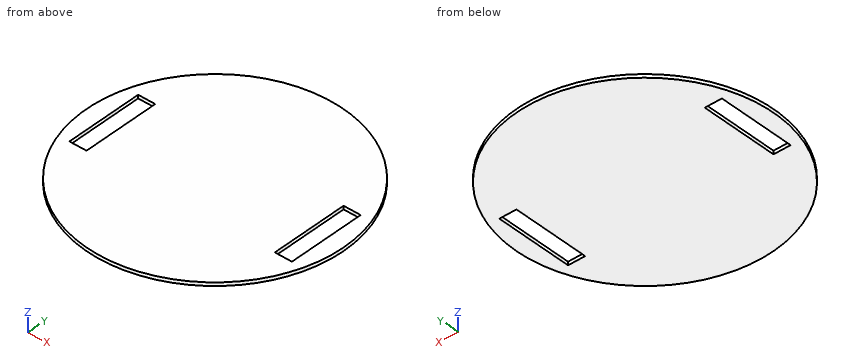
```python
from build123d import *

# Parameters (mm, degrees)
F0_R     = 75
F1_DEPTH = 2
F3_W     = 10
F3_H     = 22.5
F3_H_2   = 45
F4_DEPTH = 25


with BuildPart() as f1:
    # F0 (on Top) → F1 (new body)
    with BuildSketch(Plane.XY):
        Circle(F0_R)
    extrude(amount=F1_DEPTH)

    # F3 (on face) → F4 (cut)
    with BuildSketch(Plane.XY.offset(2)):
        with Locations((-60, -11.25)):
            Rectangle(F3_W, F3_H)
        with Locations((-60, 11.25)):
            Rectangle(F3_W, F3_H)
        with Locations((60, 0)):
            Rectangle(F3_W, F3_H_2)
    extrude(amount=-F4_DEPTH, mode=Mode.SUBTRACT)


solid = f1.part
```
Geometry check sheet. Reference: the model listing, model coordinates, mm. Coordinates: 2 decimals unless noted, no trailing zeros. Order: outer loops, then holes, each group sorted by start corner. A loop starts at its lowest first (then second) coordinate and runs counter-clockwise, first axis right, second up. Notation, with made-up numbers: (23, 60.25) - (33, 60.25) arc R16 ccw to (33, 84.25) - close; hole circle Ø1 at (75.5, 56). An arc over 180 degrees is marked (long way). Answer in a Markdown table with one row per item. Add a question column.
1. Section check D-D (x = 49). Enter the section's corners in (y, z), plus the area to 3 significant figures.
2. Material ranges on L1, parallel to X at y = -18.5, z = 0.9; L2, parallel to X at y = -19.5, z = 0.3; L3, parallel to Y at x = -64, z = 1.5, recorded low to high. Write a range as [from, to].
3. Gauge pin test, flat ends, axial feed: pin 1 Ø5 at (x, y) = (14.5, -37) entering from -Z; pin 2 Ø1 at (y, z) = (-3, 1) entering from -X; pin 3 Ø1 at (y, z) = (11, 1) entering from +X; pin 4 Ø6 at (x, y) = (-59, -52) entering from +Z. Record the tip position at first contact, or that the pin passes through.
4. Section check A-A (z = 0.6). Enter the section's corners in (x, y), plus the area to 3 significant figures.
5. Section check B-B (y = 0). Enter the section's corners in (x, z).
6. Section check C-C (y = -18). Enter the section's corners in (x, z).
Data:
| question | item | result |
|---|---|---|
| 1 | outline | (-56.78, 0) - (56.78, 0) - (56.78, 2) - (-56.78, 2) - close |
| 1 | area | 227 mm² |
| 2 | L1 | x = [-72.68, -65], [-55, 55], [65, 72.68] |
| 2 | L2 | x = [-72.42, -65], [-55, 55], [65, 72.42] |
| 2 | L3 | y = [-39.1, -22.5], [22.5, 39.1] |
| 3 | pin 1 | stops at z = 0 |
| 3 | pin 2 | stops at x = -74.96 |
| 3 | pin 3 | stops at x = 74.26 |
| 3 | pin 4 | passes through |
| 4 | outline | circle Ø150 at (0, 0); hole (-65, -22.5) - (-55, -22.5) - (-55, 22.5) - (-65, 22.5) - close; hole (55, -22.5) - (65, -22.5) - (65, 22.5) - (55, 22.5) - close |
| 4 | area | 16,800 mm² |
| 5 | outline | (-75, 0) - (-65, 0) - (-65, 2) - (-75, 2) - close; (-55, 0) - (55, 0) - (55, 2) - (-55, 2) - close; (65, 0) - (75, 0) - (75, 2) - (65, 2) - close |
| 6 | outline | (-72.81, 0) - (-65, 0) - (-65, 2) - (-72.81, 2) - close; (-55, 0) - (55, 0) - (55, 2) - (-55, 2) - close; (65, 0) - (72.81, 0) - (72.81, 2) - (65, 2) - close |
